Model file for the job. Use its own axes, mm. Coordinates: 2 decimals unless noted, no trailing zeros. Write each loop counter-clockwise with the first axis right and the second up, starting at its lowest first coordinate (ties: lowest second). Pieces come first, ordered by that corner, then holes.
Q1. Band-saw the part on D-D, the plane x = 60. Write the cut outline in (y, z).
Q2. Band-saw the part on A-A, the plane z = 35. Write the cut outline in (x, y).
Q3. Drill centre lines: probe 1 along X at (y, z) = (0.6, 20); probe 2 along X at (y, z) = (1.8, 35). Where is each one in solid material? Low to high.
Q4. Band-saw the part on C-C, the plane z = 20. Write the cut outline in (x, y).
Q5. Band-saw the part on B-B, the plane x = 15. Write the cut outline in (y, z).
Q6. Pin check, flat tip, straight feed: P1, Ø1.9, axis at x = 5, z = 20, coming from the +Y side. Stop position of the tip, or through.
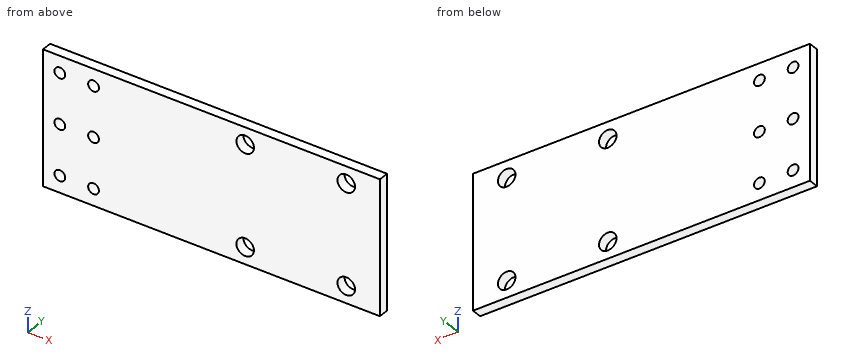
from build123d import *

# Parameters (mm, degrees)
SKETCH_1_W          = 100
SKETCH_1_H          = 40
SKETCH_1_R          = 1.6
EXTRUDE_1_DEPTH     = 3
SKETCH_2_R          = 2.6
CUT_EXTRUDE_1_DEPTH = 3


with BuildPart() as part:
    # 草图1 → 凸台-拉伸1 (new body)
    with BuildSketch(Plane(origin=(0, 0, 0), x_dir=(1, 0, 0), z_dir=(0, 1, 0))):
        with Locations((50, -20)):
            Rectangle(SKETCH_1_W, SKETCH_1_H)
        with Locations(Location((5, -20, 0), (0, 0, 270))):
            Circle(SKETCH_1_R, mode=Mode.SUBTRACT)
        with Locations(Location((5, -5, 0), (0, 0, 270))):
            Circle(SKETCH_1_R, mode=Mode.SUBTRACT)
        with Locations(Location((15, -20, 0), (0, 0, 90))):
            Circle(SKETCH_1_R, mode=Mode.SUBTRACT)
        with Locations(Location((15, -5, 0), (0, 0, 90))):
            Circle(SKETCH_1_R, mode=Mode.SUBTRACT)
        with Locations(Location((15, -35, 0), (0, 0, 270))):
            Circle(SKETCH_1_R, mode=Mode.SUBTRACT)
        with Locations(Location((5, -35, 0), (0, 0, 90))):
            Circle(SKETCH_1_R, mode=Mode.SUBTRACT)
    extrude(amount=EXTRUDE_1_DEPTH)

    # 草图2 → 切除-拉伸1 (cut)
    with BuildSketch(Plane(origin=(0, 3, 0), x_dir=(1, 0, 0), z_dir=(0, 1, 0))):
        with Locations(Location((60, -5, 0), (0, 0, 270))):
            Circle(SKETCH_2_R)
        with Locations(Location((60, -35, 0), (0, 0, 90))):
            Circle(SKETCH_2_R)
        with Locations(Location((90, -35, 0), (0, 0, 270))):
            Circle(SKETCH_2_R)
        with Locations(Location((90, -5, 0), (0, 0, 90))):
            Circle(SKETCH_2_R)
    extrude(amount=-CUT_EXTRUDE_1_DEPTH, mode=Mode.SUBTRACT)


solid = part.part
Answer sheet:
1. outline: (0, 0) - (3, 0) - (3, 2.4) - (0, 2.4) - close; (0, 7.6) - (3, 7.6) - (3, 32.4) - (0, 32.4) - close; (0, 37.6) - (3, 37.6) - (3, 40) - (0, 40) - close
2. outline: (0, 0) - (3.4, 0) - (3.4, 3) - (0, 3) - close; (6.6, 0) - (13.4, 0) - (13.4, 3) - (6.6, 3) - close; (16.6, 0) - (57.4, 0) - (57.4, 3) - (16.6, 3) - close; (62.6, 0) - (87.4, 0) - (87.4, 3) - (62.6, 3) - close; (92.6, 0) - (100, 0) - (100, 3) - (92.6, 3) - close
3. probe 1: x = 0 to 3.4, 6.6 to 13.4, 16.6 to 100
3. probe 2: x = 0 to 3.4, 6.6 to 13.4, 16.6 to 57.4, 62.6 to 87.4, 92.6 to 100
4. outline: (0, 0) - (3.4, 0) - (3.4, 3) - (0, 3) - close; (6.6, 0) - (13.4, 0) - (13.4, 3) - (6.6, 3) - close; (16.6, 0) - (100, 0) - (100, 3) - (16.6, 3) - close
5. outline: (0, 0) - (3, 0) - (3, 3.4) - (0, 3.4) - close; (0, 6.6) - (3, 6.6) - (3, 18.4) - (0, 18.4) - close; (0, 21.6) - (3, 21.6) - (3, 33.4) - (0, 33.4) - close; (0, 36.6) - (3, 36.6) - (3, 40) - (0, 40) - close
6. P1: passes through
